CAD build for the part. Positions are in the model's coordinates, mm. A direction names the side the tool comes from. Coordinates: 2 decimals unless noted, no trailing zeros. Loops run counter-clockwise (first coordinate to the right, second up) from the corner with the lowest first, then second, coordinate; pieces in that order, holes last.
1) Pin check, flat tips, straight feed: pin 1 Ø2 at (y, z) = (5, -196) entering from -X; pin 2 Ø2.5 at (y, z) = (3.5, -34) entering from -X. Stop position of each tip, or through.
2) Saw through at A-A, the plane x = -3.25. Write the cut outline in (y, z), and give its area (3 significant figures).
3) Wall check: line 1 along Y through (x, z) = (1.8, -34); line 2 along X through (y, z) = (0.5, -185.5); line 3 along Z through (x, y) = (-6, 2.5). Give the ranges that are in metal, low to high.
4) Which spindle directions (+Z, -Z, +X, -X, +Y, -Y) get a long thin tool onto all of the face, cutting with end or side? Do faces 1 (the flat face through (-10, 4, -397)), 2 (the flat face through (4, 4, -201)). Say none if no direction does.
5) Saw through at B-B, the plane z = -140.5. Write the cut outline in (x, y).
```python
from build123d import *

# Parameters (mm, degrees)
SKETCH_1_R      = 1.5
EXTRUDE_1_DEPTH = 4
SKETCH_2_W      = 20
SKETCH_2_H      = 7
EXTRUDE_2_DEPTH = 3


with BuildPart() as part:
    # 草图1 → 凸台-拉伸1 (new body)
    with BuildSketch(Plane(origin=(0, 0, 0), x_dir=(0, 0, -1), z_dir=(1, 0, 0))):
        with BuildLine():
            Line((400, 7), (400, 0))
            Line((400, 0), (0, 0))
            ThreePointArc((0, 0), (-3.5, 3.5), (0, 7))
            Line((0, 7), (400, 7))
        make_face()
        with Locations((0, 3.5)):
            Circle(SKETCH_1_R, mode=Mode.SUBTRACT)
        with Locations((34, 3.5)):
            Circle(SKETCH_1_R, mode=Mode.SUBTRACT)
    extrude(amount=EXTRUDE_1_DEPTH)

    # 草图2 → 凸台-拉伸2 (add)
    with BuildSketch(Plane(origin=(0, 0, -400), x_dir=(-1, 0, 0), z_dir=(0, 0, -1))):
        with Locations((10, 3.5)):
            Rectangle(SKETCH_2_W, SKETCH_2_H)
    extrude(amount=-EXTRUDE_2_DEPTH)


solid = part.part
```
Data:
1. pin 1: stops at x = 0
1. pin 2: passes through
2. outline: (0, -400) - (7, -400) - (7, -397) - (0, -397) - close
2. area: 21.0 mm2
3. line 1: y = 0 to 2, 5 to 7
3. line 2: x = 0 to 4
3. line 3: z = -400 to -397
4. face 1: +Z, -X, +Y, -Y
4. face 2: +Z, -Z, +X, +Y, -Y
5. outline: (0, 0) - (4, 0) - (4, 7) - (0, 7) - close
